Read the model definition and answer for the solid it produces. Units are mm, in the model's axes. Face numbers are marked on the shaded views. A direction names the side the tool comes from. Coordinates: 2 decimals unless noted, no trailing zeros. Loops run counter-clockwise (first coordinate to the right, second up) from the corner with the lowest first, then second, coordinate; pieces in that order, holes last. Notation, with made-up numbers: M -11.5,48.25 L 19.5,48.25 A33 ccw 19.5,86.25 Z; hole C 32,-29 d5. An arc over 180 degrees is marked long. Put each result on its own line as item: value.
Autodesk Inventor part; units mm, degrees
ref_plane "YZ Plane" through (0, 0, 0) normal (1, 0, 0) x (0, 1, 0)
ref_plane "XZ Plane" through (0, 0, 0) normal (0, 1, 0) x (-1, 0, 0)
ref_plane "XY Plane" through (0, 0, 0) normal (0, 0, 1) x (1, 0, 0)
sketch "Sketch1" plane through (0, 0, 0) normal (0, 0, 1) x (1, 0, 0)
  line L0 (0, 0) -> (-22, 0)
  line L1 (-22, 0) -> (-22, 0)
  line L2 (-22, 0) -> (-14.5, 0)
  line L3 (-22, 0) -> (-22, 25.4)
  line L4 (-22, 25.4) -> (0, 25.4)
  line L5 (-29.0722, -4.6) -> (-18.7593, -4.6) construction
  line L6 (-22, 0) -> (0, 0) construction
  line L7 (0, 0) -> (22, 0) construction
  line L8 (0, -10.6) -> (0, 31.4) construction
  line L9 (0, -4.6) -> (0, 12.9) construction
  line L10 (0, -4.6) -> (-10, -4.6) construction
  line L11 (0, -4.6) -> (10, -4.6) construction
  line L12 (-10, -4.6) -> (-10, 0) construction
  line L13 (-10, 0) -> (-6.1, 3.9) construction
  line L14 (-6.1, 3.9) -> (-6.1, 4.4) construction
  line L15 (-6.1, 4.4) -> (-10, 8.3) construction
  line L16 (-10, 8.3) -> (-10, 10.8) construction
  line L17 (-10, 10.8) -> (-7.9, 12.9) construction
  line L18 (-7.9, 12.9) -> (0, 12.9) construction
  line L19 (10, 0) -> (6.1, 3.9) construction
  line L20 (6.1, 3.9) -> (6.1, 4.4) construction
  line L21 (6.1, 4.4) -> (10, 8.3) construction
  line L22 (10, 8.3) -> (10, 10.8) construction
  line L23 (10, 10.8) -> (7.9, 12.9) construction
  line L24 (10, -4.6) -> (10, 0) construction
  line L25 (7.9, 12.9) -> (0, 12.9) construction
  line L26 (-14.5, 8.3) -> (-14.5, 10.8)
  line L27 (-14.5, 10.8) -> (-7.9, 17.4)
  line L28 (-7.9, 17.4) -> (0, 17.4)
  line L29 (-14.5, 0) -> (-10.6, 3.9)
  line L30 (-10.6, 3.9) -> (-10.6, 4.4)
  line L31 (-10.6, 4.4) -> (-14.5, 8.3)
  line L32 (-10.6, 3.9) -> (-6.1, 3.9) construction
  line L33 (-10, 8.3) -> (-14.5, 8.3) construction
  line L34 (22, 0) -> (14.5, 0)
  line L35 (22, 0) -> (22, 25.4)
  line L36 (22, 25.4) -> (0, 25.4)
  line L37 (14.5, 8.3) -> (14.5, 10.8)
  line L38 (14.5, 10.8) -> (7.9, 17.4)
  line L39 (7.9, 17.4) -> (0, 17.4)
  line L40 (14.5, 0) -> (10.6, 3.9)
  line L41 (10.6, 3.9) -> (10.6, 4.4)
  line L42 (10.6, 4.4) -> (14.5, 8.3)
  point P0 (-3.95, 17.4)
  dimension "d0" = 4.6
  dimension "d1" = 44
  dimension "d3" = 17.5
  dimension "d4" = 20
  dimension "d5" = 4.6
  dimension "d6" = 8.5
  dimension "d7" = 135
  dimension "d8" = 0.5
  dimension "d9" = 135
  dimension "d10" = 2.5
  dimension "d11" = 7.5
  dimension "d12" = 25.4
  dimension "d13" = 45
  dimension "d14" = 135
  dimension "d15" = 2.5
  dimension "d16" = 0.5
  dimension "d17" = 135
  dimension "d19" = 4.5
extrude "Extrusion1" add sketch "Sketch1" along normal blind 77.5
sketch "Sketch2" plane through (-22, 25.4, 0) normal (0, 1, 0) x (1, 0, 0)
  circle A0 centre (6, -20.75) radius 2
  circle A1 centre (6, -56.75) radius 2
  line L0 (6, -20.75) -> (6, -56.75)
  circle A2 centre (38, -20.75) radius 2
  circle A3 centre (38, -56.75) radius 2
  line L1 (38, -20.75) -> (38, -56.75) construction
  line L2 (22, 0) -> (22, -77.5) construction
  line L3 (44, -77.5) -> (0, -77.5) construction
  line L4 (38, -38.75) -> (22, -38.75) construction
  line L5 (6, -38.75) -> (22, -38.75) construction
  line L6 (0, 0) -> (0, -77.5) construction
  line L7 (44, -64) -> (0, -64) construction
  line L8 (0, -64) -> (0, -13.5) construction
  line L9 (0, -13.5) -> (44, -13.5) construction
  line L10 (44, -13.5) -> (44, -64) construction
  line L11 (44, -64) -> (0, -13.5) construction
  line L12 (0, -64) -> (44, -13.5) construction
  line L13 (44, 0) -> (44, -77.5)
  line L14 (0, -13.5) -> (44, -13.5)
  line L15 (44, -13.5) -> (44, 0)
  line L16 (44, 0) -> (0, 0)
  line L17 (0, 0) -> (0, -13.5)
  line L18 (0, -64) -> (44, -64)
  line L19 (44, -64) -> (44, -77.5)
  line L20 (44, -77.5) -> (0, -77.5)
  line L21 (0, -77.5) -> (0, -64)
  point P0 (7.5, -77.5)
  dimension "d22" = 36
  dimension "d23" = 4
  dimension "d24" = 4
  dimension "d25" = 36
  dimension "d26" = 4
  dimension "d27" = 4
  dimension "d29" = 32
  dimension "d30" = 50.5
extrude "Extrusion2" cut sketch "Sketch2" against normal blind 8 contours A0 | A1 | A2 | A3
extrude "Extrusion3" cut sketch "Sketch2" against normal blind 4 contours L13 L20 L21 L18 | L13 L14 L17 L16
sketch "Sketch3" plane through (22, 0, 77.5) normal (1, 0, 0) x (0, 0, -1)
  circle A0 centre (7.5, 14.4) radius 2
  circle A1 centre (70, 14.4) radius 2
  line L0 (64, 21.4) -> (64, 25.4)
  line L1 (13.5, 25.4) -> (13.5, 21.4)
  line L2 (13.5, 21.4) -> (0, 21.4)
  line L3 (77.5, 21.4) -> (64, 21.4)
  point P0 (77.5, 0)
  point P1 (64, 23.4)
  dimension "d35" = 6
  dimension "d36" = 6
  dimension "d37" = 7
  dimension "d38" = 7
  dimension "d39" = 4
  dimension "d40" = 4
extrude "Extrusion4" cut sketch "Sketch3" against normal blind 5
mirror "Mirror1" about plane through (0, 0, 0) normal (1, 0, 0) of "Extrusion4"
equation "\"d15\" = d10"
equation "\"d16\" = d8"
properties part number "HGH20CA Slider Block"
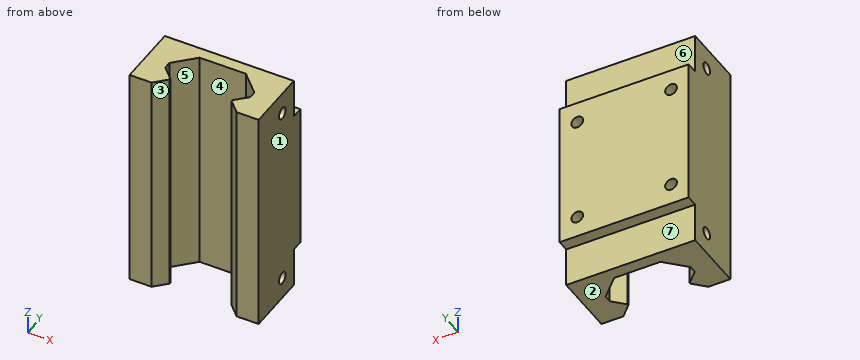
1) Straight lines are drawn through the part: line 1 (X direction, y = 19.5, z = 20.75); line 2 (Z direction, x = 15, y = 17.5); line 3 (Y direction, x = -20.95, z = 7.5). For each, find the intervals that lie inside material, in ascending order. Write a range as [from, to].
Answer list:
line 1: x = [-22, -18], [-14, 14], [18, 22]
line 2: z = [0, 19.02], [22.48, 55.02], [58.48, 77.5]
line 3: y = [0, 12.4], [16.4, 21.4]
2) Find section D-D, the plane x = -12.5. Write down the section's boundary in (y, z), plus the area to 3 significant figures.
Answer list:
outline: M 2,0 L 6.3,0 L 6.3,77.5 L 2,77.5 Z; M 12.8,0 L 21.4,0 L 21.4,13.5 L 25.4,13.5 L 25.4,64 L 21.4,64 L 21.4,77.5 L 12.8,77.5 Z
area: 1,200 mm^2
3) Find section C-C, the plane z = 17.5. Write down the section's boundary in (x, y).
Answer list:
outline: M -22,0 L -14.5,0 L -10.6,3.9 L -10.6,4.4 L -14.5,8.3 L -14.5,10.8 L -7.9,17.4 L 7.9,17.4 L 14.5,10.8 L 14.5,8.3 L 10.6,4.4 L 10.6,3.9 L 14.5,0 L 22,0 L 22,25.4 L -22,25.4 Z
4) Find section B-B, the plane y = 7. Write down the section's boundary in (x, z).
Answer list:
outline: M -22,0 L -13.2,0 L -13.2,77.5 L -22,77.5 Z; M 13.2,0 L 22,0 L 22,77.5 L 13.2,77.5 Z
5) Determine the mould class of the marked faces 1, 2, 3 and 4 for opening direction X: released by +X, released by -X, zero draft, split by the parting line, or undercut.
Answer list:
face 1: released by +X
face 2: zero draft
face 3: undercut
face 4: undercut
6) Given pin 1 Ø4.5 at (y, z) = (14.4, 70) entering from +X; pin 2 Ø2 at (x, z) = (-16.5, 20.5) entering from +Y; pin 3 Ø1.2 at (y, z) = (15.5, 70) entering from +X; pin 4 Ø3 at (y, z) = (14, 70) entering from -X, each flat-ended and moving along its own axis, determine where each tip first touches the part or whether it passes through.
Answer list:
pin 1: stops at x = 22
pin 2: stops at y = 17.4
pin 3: stops at x = 17
pin 4: stops at x = -17
7) Find section A-A, the plane x = 13. Write down the section's boundary in (y, z).
Answer list:
outline: M 1.5,0 L 6.8,0 L 6.8,77.5 L 1.5,77.5 Z; M 12.3,0 L 21.4,0 L 21.4,13.5 L 25.4,13.5 L 25.4,64 L 21.4,64 L 21.4,77.5 L 12.3,77.5 Z
8) Which of the six approach directions +Z, -Z, +X, -X, +Y, -Y give full straight-line access (tool end or side, diameter ignored) to the marked faces 5, 6 and 7?
Answer list:
face 5: +Z, -Z
face 6: +Z, +X, -X, +Y
face 7: -Z, +X, -X, +Y
